The figure shows three views and two pictorial views of one solid part (mm, origin at its lowest corner). Answer the questions. Give positions to 0.01 mm unless a question says otherwise; leave off trailing zeros. Order: outer loops, then holes, each group sorted by start corner. A loop starts at its lowest first (then second) coordinate and runs counter-clockwise, first axis right, second up. Notation, with made-up numbers: (-34, 24) - (-30, 24) arc R5 ccw to (-30, 29) - close; hole circle Ø1 at (17.5, 80). An arc over 180 degrees is marked (long way). Answer as a JSON object with one key per item and string values. Group by question number.
Q1. Consider line 1 (X direction, y = 93.5, z = 6); line 2 (Z direction, x = 66.5, y = 5); line 3 (X direction, y = 74, z = 46). Determine where each line is inside the solid, lowest interval first.
Q2. Given pin 1 (12 mm diameter, centred on x = 51.5, y = 25, fed in from -Z), flat-ended and moving along its own axis, determine where the tip first touches the part or whether it passes through.
Q3. A cutting plane is placed at A-A, the plane z = 46. Give the vertices of the cut face in (x, y) (3 decimals), and give its area (3 significant figures).
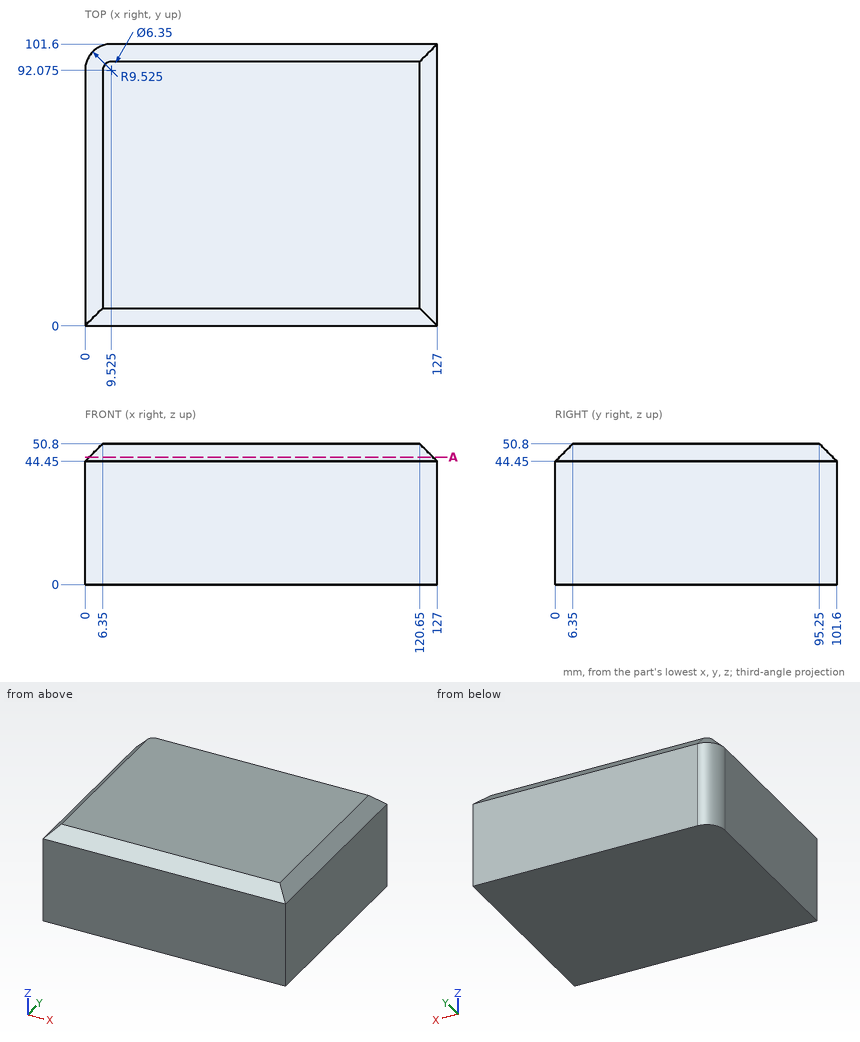
Reply:
{
 "1": {"line 1": "x = 0.11 to 127", "line 2": "z = 0 to 49.45", "line 3": "x = 1.55 to 125.45"},
 "2": {"pin 1": "stops at z = 0"},
 "3": {"outline": "(1.55, 1.55) - (125.45, 1.55) - (125.45, 100.05) - (9.525, 100.05) arc R7.975 ccw to (1.55, 92.075) - close", "area": "12,200 mm^2"}
}
